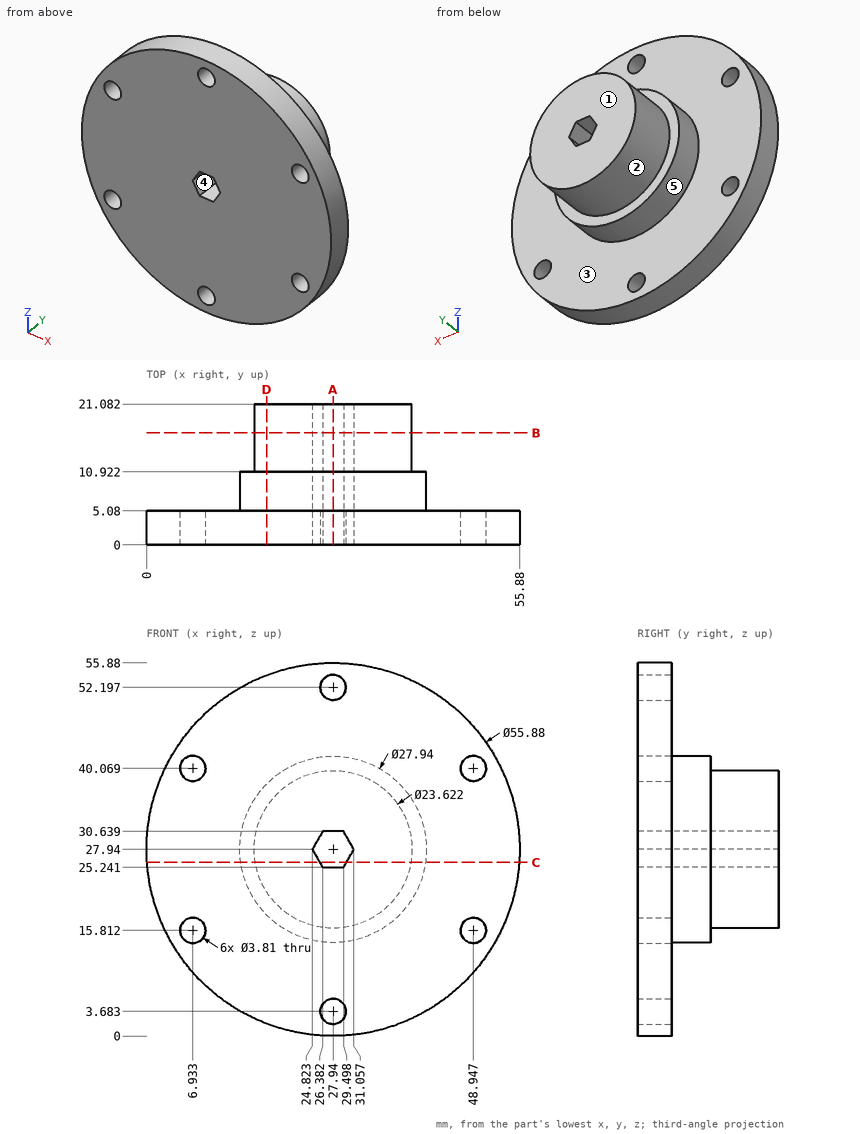
Drawing for the job (mm, zero at the part's lowest x, y, z). A direction names the side the tool comes from. Round coordinates to 2 decimals unless told otherwise and drop trailing zeros. Loops run counter-clockwise (first coordinate to the right, second up) from the corner with the lowest first, then second, coordinate; pieces in that order, holes last. Notation, with made-up numbers: M 22,27 L 50,27 A7 cw 50,34 Z; hole C 30.25,75 d11. An arc over 180 degrees is marked long. Use a Markdown table: item, result. Add a question column.
(1) Drill centre lines: line 1 (Z direction, x = 27.94, y = 4.05); line 2 (Z direction, x = 27.5, y = 20); line 3 (Y direction, x = 43.5, z = 28). Where is each one in solid material? Low to high.
(2) Flat gauge pins, fed straight in: pin 1 (10 mm diameter, centred on x = 46.5, y = 16.5, fed in from -Z); pin 2 (5 mm diameter, centred on x = 39.5, y = 15, fed in from +Z); pin 3 (0.9 mm diameter, centred on x = 28, y = 12, fed in from -Z); pin 4 (3 mm diameter, centred on y = 18, z = 32.5, fed in from +X). Where does each tip first touch, or does it go through?
(3) Cut at A-A (x = 27.94). Give the cut face in (y, z).
(4) Cut at B-B (y = 16.75). Give the cut face in (x, z), and give its area (3 significant figures).
(5) Pull direction Z, two halves, no side cores. Call the marked faces 3, 4 and 5: +Z half, -Z half, draft (parallel to the pull), parting line (faces both ways), or undercut.
(6) Cut at C-C (z = 26). Give the cut face in (x, y) (1 decimal).
(7) Cut at D-D (x = 18). Give the cut face in (y, z).
(8) Which spindle directions (+Z, -Z, +X, -X, +Y, -Y) get a long thin tool onto all of the face, cutting with end or side? Do the marked faces 1 and 2. Say none if no direction does.
Geometry says:
| question | item | result |
|---|---|---|
| 1 | line 1 | z = 0 to 1.78, 5.59 to 25.24, 30.64 to 50.29, 54.1 to 55.88 |
| 1 | line 2 | z = 16.14 to 25.24, 30.64 to 39.74 |
| 1 | line 3 | y = 0 to 5.08 |
| 2 | pin 1 | passes through |
| 2 | pin 2 | stops at z = 35.52 |
| 2 | pin 3 | stops at z = 16.13 |
| 2 | pin 4 | stops at x = 39.35 |
| 3 | outline | M 0,0 L 5.08,0 L 5.08,1.78 L 0,1.78 Z; M 0,5.59 L 5.08,5.59 L 5.08,13.97 L 10.92,13.97 L 10.92,16.13 L 21.08,16.13 L 21.08,25.24 L 0,25.24 Z; M 0,30.64 L 21.08,30.64 L 21.08,39.75 L 10.92,39.75 L 10.92,41.91 L 5.08,41.91 L 5.08,50.29 L 0,50.29 Z; M 0,54.1 L 5.08,54.1 L 5.08,55.88 L 0,55.88 Z |
| 4 | outline | C 27.94,27.94 d23.62; hole M 24.82,27.94 L 26.38,25.24 L 29.5,25.24 L 31.06,27.94 L 29.5,30.64 L 26.38,30.64 Z |
| 4 | area | 413 mm² |
| 5 | face 3 | draft |
| 5 | face 4 | undercut |
| 5 | face 5 | parting line |
| 6 | outline | M 0.1,0 L 25.9,0 L 25.9,21.1 L 16.3,21.1 L 16.3,10.9 L 14.1,10.9 L 14.1,5.1 L 0.1,5.1 Z; M 29.9,0 L 55.8,0 L 55.8,5.1 L 41.8,5.1 L 41.8,10.9 L 39.6,10.9 L 39.6,21.1 L 29.9,21.1 Z |
| 7 | outline | M 0,1.83 L 5.08,1.83 L 5.08,18.12 L 10.92,18.12 L 10.92,21.56 L 21.08,21.56 L 21.08,34.32 L 10.92,34.32 L 10.92,37.76 L 5.08,37.76 L 5.08,54.05 L 0,54.05 Z |
| 8 | face 1 | +Z, -Z, +X, -X, +Y |
| 8 | face 2 | +Y |
